Geometry: final body of the model. Coordinates: model frame, mm. Face numbers are marked on the shaded views. A direction names the side the tool comes from. Give positions to 0.01 mm unless a question says otherwise; leave off trailing zeros. Loops run counter-clockwise (first coordinate to the right, second up) from the corner with the lowest first, then second, coordinate; pieces in that order, holes last.
1. Section A-A, the plane z = 10.25. Output: boundary loops of the cut face in (x, y), then the cut area to 3 significant figures.
2. Access query for the marked faces 1 and 2. Directions: +Z, -Z, +X, -X, +Y, -Y. A direction counts if a zero-diameter tool reaches every point of the face in a straight line with its end or side. Return the directions, or none.
3. Section D-D, the plane z = -6.25. Output: boundary loops of the cut face in (x, y).
4. Section B-B, the plane y = 0.75. Output: boundary loops of the cut face in (x, z).
5. Section C-C, the plane x = -0.25. Output: boundary loops of the cut face in (y, z).
6. Material intervals for line 1 along Y through (x, z) = (-1, -5); line 2 along X through (y, z) = (1.25, 2.75); line 3 along Y through (x, z) = (1.5, 11.5), sorted ascending.
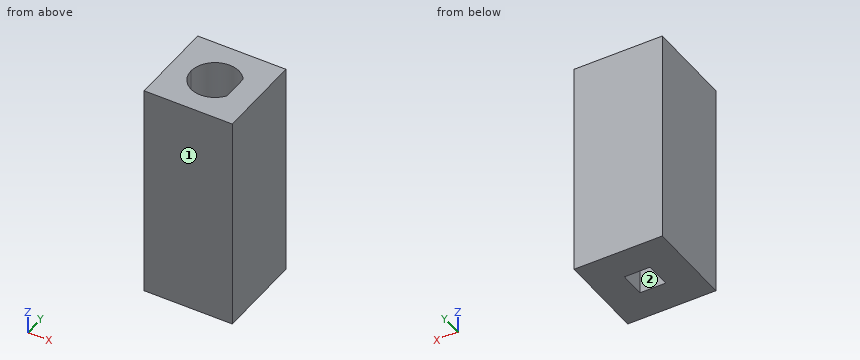
from build123d import *

# Parameters (mm, degrees)
F0_W     = 11
F0_H     = 11
F1_DEPTH = 14.2
F2_W     = 11
F2_H     = 11
F3_DEPTH = 3
F4_W     = 11
F4_H     = 11
F4_W_2   = 3.2
F4_H_2   = 3.2
F5_DEPTH = 10
F6_DEPTH = 25


# Not quite as in the source:
# - a feature names something its author has since deleted; it is built from what else it names


with BuildPart() as f1:
    # F0 (on Top) → F1 (new body)
    with BuildSketch(Plane.XY):
        Rectangle(F0_W, F0_H)
        with BuildLine():
            ThreePointArc((2.5, 1.6583123952), (2.8722813233, 0.8660254038), (3, 0))
            ThreePointArc((3, 0), (2.8722813233, -0.8660254038), (2.5, -1.6583123952))
            ThreePointArc((2.5, -1.6583123952), (-0.8660254038, -2.8722813233), (-3, 0))
            ThreePointArc((-3, 0), (-0.8660254038, 2.8722813233), (2.5, 1.6583123952))
        make_face(mode=Mode.SUBTRACT)
        with BuildLine():
            ThreePointArc((2.5, -1.6583123952), (2.8722813233, -0.8660254038), (3, 0))
            ThreePointArc((3, 0), (2.8722813233, 0.8660254038), (2.5, 1.6583123952))
            Line((2.5, 1.6583123952), (2.5, 0))
            Line((2.5, 0), (2.5, -1.6583123952))
        make_face()
    extrude(amount=F1_DEPTH)

    # F2 (on face) → F3 (join)
    with BuildSketch(Plane(origin=(0, 0, 0), x_dir=(1, 0, 0), z_dir=(0, 0, -1))):
        Rectangle(F2_W, F2_H)
        with BuildLine():
            ThreePointArc((2.5, -1.6583123952), (-3, 0), (2.5, 1.6583123952))
            Line((2.5, 1.6583123952), (2.5, -1.6583123952))
        make_face(mode=Mode.SUBTRACT)
        with BuildLine():
            Line((2.5, -1.6583123952), (2.5, 1.6583123952))
            ThreePointArc((2.5, 1.6583123952), (-3, 0), (2.5, -1.6583123952))
        make_face()
    extrude(amount=F3_DEPTH)

    # F4 (on face) → F5 (join)
    with BuildSketch(Plane(origin=(0, 0, -3), x_dir=(1, 0, 0), z_dir=(0, 0, -1))):
        Rectangle(F4_W, F4_H)
        Rectangle(F4_W_2, F4_H_2, mode=Mode.SUBTRACT)
    extrude(amount=F5_DEPTH)

    # F6 (cut): a face of the model
    f6_faces = [f1.faces().sort_by_distance(p)[0] for p in [
        (0, 0, -3),
    ]]
    extrude(f6_faces, amount=-F6_DEPTH, mode=Mode.SUBTRACT)


solid = f1.part
Answers below:
1. outline: (-5.5, -5.5) - (5.5, -5.5) - (5.5, 5.5) - (-5.5, 5.5) - close; hole (2.5, -1.66) - (2.5, 1.66) arc R3 ccw (long way) to start
1. area: 93.9 mm2
2. face 1: +Z, -Z, +X, -X, -Y
2. face 2: +Z, -Z
3. outline: (-5.5, -5.5) - (5.5, -5.5) - (5.5, 5.5) - (-5.5, 5.5) - close; hole (-1.6, -1.6) - (1.6, -1.6) - (1.6, 1.6) - (-1.6, 1.6) - close
4. outline: (-5.5, -13) - (-1.6, -13) - (-1.6, 0) - (-2.9, 0) - (-2.9, 14.2) - (-5.5, 14.2) - close; (1.6, -13) - (5.5, -13) - (5.5, 14.2) - (2.5, 14.2) - (2.5, 0) - (1.6, 0) - close
5. outline: (-5.5, -13) - (-1.6, -13) - (-1.6, 0) - (-2.99, 0) - (-2.99, 14.2) - (-5.5, 14.2) - close; (1.6, -13) - (5.5, -13) - (5.5, 14.2) - (2.99, 14.2) - (2.99, 0) - (1.6, 0) - close
6. line 1: y = -5.5 to -1.6, 1.6 to 5.5
6. line 2: x = -5.5 to -2.73, 2.5 to 5.5
6. line 3: y = -5.5 to -2.6, 2.6 to 5.5
